Solid Edge part; units mm, degrees
sketch "Sketch1" plane through (0, 0, 0) normal (0, 0, 1) x (1, 0, 0)
  line L0 (-142.255, -41.9) -> (142.255, -41.9)
  line L1 (142.255, -41.9) -> (142.255, 41.9)
  line L2 (142.255, 41.9) -> (-142.255, 41.9)
  line L3 (-142.255, 41.9) -> (-142.255, -41.9)
extrude "Protrusion1" add sketch "Sketch1" against normal blind 20
sketch "Sketch2" plane through (0, 0, 0) normal (0, 0, 1) x (0, 1, 0)
  circle A0 centre (-6.6, -81.075) radius 6.5
  circle A1 centre (-11.6, -177.075) radius 60
extrude "ExtrudedCutout_1" cut sketch "Sketch2" against normal blind 20
fillet "Round_1" radius 3 2 edges at (125.2878, -41.9, -10) (142.255, 41.9, -10)
Could you check a few things on this model? Use its own coordinates, in mm. Round coordinates to 2 decimals unless told otherwise and drop trailing zeros. Order: outer loops, then holes, each group sorted by start corner. A loop starts at its lowest first (then second) coordinate and runs counter-clockwise, first axis right, second up. Notation, with made-up numbers: M -28,52 L -11,52 A28 cw -11,91 Z; hole C 81.25,78 d1. An arc over 180 degrees is marked long. One line per item, written item: value.
(1) Imagine slicing it at A-A (y = -6.6). Write out the boundary of the cut face in (x, z) (3 decimals).
Ans:
outline: M -142.255,-20 L 74.575,-20 L 74.575,0 L -142.255,0 Z; M 87.575,-20 L 117.284,-20 L 117.284,0 L 87.575,0 Z
(2) I need wall thicknesses on line 1 along X through (y, z) = (35, -3.75) (3 decimals); line 2 along X through (y, z) = (-6.6, -7.5) (3 decimals); line 3 along Y through (x, z) = (87, -3.5). Which ranges of each line are inside material? Lowest first, please. Write a range as from..to.
Ans:
line 1: x = -142.255..139.28
line 2: x = -142.255..74.575, 87.575..117.284
line 3: y = -41.9..-9.27, -3.93..41.9
(3) I'm going to push flat-ended pins straight in: P1, Ø2, axis at y = 15, z = -15.5, coming from the +X side; P2, Ø11.5, axis at x = 81.075, y = -6.6, coming from the -Z side; P3, Ø8, axis at y = -28.5, z = -10, coming from the +X side. Where does each tip first touch, or does it pass through?
Ans:
P1: stops at x = 123.8
P2: passes through
P3: stops at x = 120.83
(4) Imagine slicing it at C-C (y = 6.5). Write out the boundary of the cut face in (x, z) (3 decimals).
Ans:
outline: M -142.255,-20 L 119.87,-20 L 119.87,0 L -142.255,0 Z
(5) If we mould it in two halves opening along X, with no side actions, what happens to faces 1 (the flat face through (-2, 1, -20)), 2 (the flat face through (-142.255, 1, -10)), 3 (the cylindrical face through (76.68, -11.39, -9.86))? For each: released by +X, released by -X, zero draft, split by the parting line, or undercut.
Ans:
face 1: zero draft
face 2: released by -X
face 3: undercut
(6) Imagine slicing it at B-B (z = -14.5). Write out the boundary of the cut face in (x, y) (3 decimals), and give its area (3 significant figures).
Ans:
outline: M -142.255,-41.9 L 120.297,-41.9 A3 ccw 123.001,-37.6 A60 cw 142.255,37.263 L 142.255,38.9 A3 ccw 139.255,41.9 L -142.255,41.9 Z; hole C 81.075,-6.6 d13
area: 22,200 mm^2
